```python
from build123d import *

# Parameters (mm, degrees)
SKETCH_2_R      = 10
SKETCH_2_R_2    = 4
EXTRUDE_1_DEPTH = 5
FILLET_1_R      = 50


with BuildPart() as part:
    # 草图1 → 旋转-薄壁1 (revolve)
    with BuildSketch(Plane.XY, mode=Mode.PRIVATE) as revolve_1_sk:
        Polygon((10, 120), (10, 50), (38.867513459, 0), (41.867513459, 0), (41.867513459, 3), (40.599564267, 3), (13, 50.803847577), (13, 120), align=None)
    revolve(revolve_1_sk.sketch.rotate(Axis((0, 0, 0), (0, 1, 0)), 90), axis=Axis((0, 0, 0), (0, 1, 0)))

    # 草图2 → 凸台-拉伸1 (add)
    with BuildSketch(Plane(origin=(0, 50, 0), x_dir=(1, 0, 0), z_dir=(0, 1, 0))):
        with Locations(Location((0, 0, 0), (0, 0, 90))):
            Circle(SKETCH_2_R)
        with Locations(Location((0, 0, 0), (0, 0, 270))):
            Circle(SKETCH_2_R_2, mode=Mode.SUBTRACT)
    extrude(amount=EXTRUDE_1_DEPTH)

    # 圆角1
    fillet_1_edges = [part.edges().sort_by_distance(p)[0] for p in [
        (0, 50.803847577, 13),
    ]]
    fillet(fillet_1_edges, radius=FILLET_1_R)


solid = part.part
```
The listing builds one solid part. Answer for the finished solid, in the listing's coordinates (mm). A direction names the side the tool comes from. Round coordinates to 2 decimals unless told otherwise and drop trailing zeros. Loops run counter-clockwise (first coordinate to the right, second up) from the corner with the lowest first, then second, coordinate; pieces in that order, holes last.
1) For a pull along Z with two mould halves and no side action, classify faces 4 (the face through (22.5, 33.4, 5)), 5 (the face through (-0.1, 55, -4.3)), 6 (the face through (-3, 3, 41)) as released by +Z, released by -Z, zero draft, split by the parting line, or undercut.
Outcome:
face 4: split by the parting line
face 5: undercut
face 6: zero draft
2) Consider line 1 (X direction, y = 84, z = 0); line 2 (X direction, y = 52.4, z = 0); line 3 (Z direction, x = 7, y = 7). Determine where each line is inside the solid, lowest interval first.
Outcome:
line 1: x = -13 to -10, 10 to 13
line 2: x = -14.41 to -4, 4 to 14.41
line 3: z = -37.64 to -34.12, 34.12 to 37.64
3) A cutting plane is placed at B-B on y = 10.5. Determine the outline of the cut face in (x, z), plus the area to 3 significant figures.
Outcome:
outline: circle Ø72.54 at (0, 0); hole circle Ø65.61 at (0, 0)
area: 752 mm2
4) Given P1, Ø6, axis at x = -1, z = 0.5, coming from the -Y side; P2, Ø3, axis at x = 3.5, z = -22.5, coming from the +Y side; P3, Ø12, axis at x = 0, z = 0, coming from the +Y side; P4, Ø6.5, axis at x = 0, z = 0, coming from the -Y side, each flat-ended and moving along its own axis, determine where each tip first touches the part or whether it passes through.
Outcome:
P1: stops at y = 50
P2: stops at y = 36.48
P3: stops at y = 55
P4: passes through
5) For faces 1 (the face through (40.87, 1.52, 9.08)), 2 (the face through (-0.1, 50, -4.3)), 3 (the face through (7.91, 92.491, 10.316)), determine the directions among +Z, -Z, +X, -X, +Y, -Y from which every point of the face is accessible in a straight line to the end or side of a thin tool.
Outcome:
face 1: +Y, -Y
face 2: -Y
face 3: +Y
6) A cutting plane is placed at A-A on y = 68. Determine the outline of the cut face in (x, z).
Outcome:
outline: circle Ø26 at (0, 0); hole circle Ø20 at (0, 0)
